```python
from build123d import *

# Parameters (mm, degrees)
CUT_EXTRUDE1_DEPTH      = 55.787705795
CUT_EXTRUDE1_DEPTH_BACK = 55.787705795
SKETCH2_R               = 11.8745
SKETCH2_R_2             = 3.175
CUT_EXTRUDE2_DEPTH      = 55.787705795
CUT_EXTRUDE2_DEPTH_BACK = 55.787705795
SKETCH3_R               = 3.175
CUT_EXTRUDE3_DEPTH      = 55.787705795
CUT_EXTRUDE3_DEPTH_BACK = 55.787705795
SKETCH4_R               = 3.175


with BuildPart() as part:
    # Sketch1 → Revolve1 (revolve)
    with BuildSketch(Plane.XY, mode=Mode.PRIVATE) as revolve1_sk:
        Polygon((0, 0), (36.5125, 0), (36.5125, 3.175), (38.1508, 3.175), (38.1508, 9.525), (0, 9.525), align=None)
    revolve(revolve1_sk.sketch.rotate(Axis((0, 0, 0), (0, 1, 0)), 90), axis=Axis((0, 0, 0), (0, 1, 0)))

    # Sketch2 → Cut-Extrude1 (cut, two sides: drawn at the far end of the back side and taken through both)
    with BuildSketch(Plane(origin=(0, 9.525, 0), x_dir=(1, 0, 0), z_dir=(0, 1, 0)).offset(-CUT_EXTRUDE1_DEPTH_BACK)):
        with Locations(Location((-12.7, 20.0152, 0), (0, 0, 270))):
            Circle(SKETCH2_R)
        with Locations(Location((12.7, 20.0152, 0), (0, 0, 270))):
            Circle(SKETCH2_R)
        with Locations(Location((0, 30.1752, 0), (0, 0, 270))):
            Circle(SKETCH2_R_2)
        with Locations(Location((0, 9.8552, 0), (0, 0, 270))):
            Circle(SKETCH2_R_2)
    extrude(amount=CUT_EXTRUDE1_DEPTH + CUT_EXTRUDE1_DEPTH_BACK, mode=Mode.SUBTRACT)

    # Sketch3 → Cut-Extrude2 (cut, two sides: drawn at the far end of the back side and taken through both)
    with BuildSketch(Plane(origin=(0, 9.525, 0), x_dir=(1, 0, 0), z_dir=(0, 1, 0)).offset(-CUT_EXTRUDE2_DEPTH_BACK)):
        with Locations(Location((-28.575, 0, 0), (0, 0, 270))):
            Circle(SKETCH3_R)
        with Locations(Location((28.575, 0, 0), (0, 0, 270))):
            Circle(SKETCH3_R)
    extrude(amount=CUT_EXTRUDE2_DEPTH + CUT_EXTRUDE2_DEPTH_BACK, mode=Mode.SUBTRACT)

    # Sketch4 → Cut-Extrude3 (cut, two sides: drawn at the far end of the back side and taken through both)
    with BuildSketch(Plane(origin=(0, 9.525, 0), x_dir=(1, 0, 0), z_dir=(0, 1, 0)).offset(-CUT_EXTRUDE3_DEPTH_BACK)):
        with Locations(Location((-15.875, -9.652, 0), (0, 0, 270))):
            Circle(SKETCH4_R)
        with Locations(Location((15.875, -9.652, 0), (0, 0, 270))):
            Circle(SKETCH4_R)
    extrude(amount=CUT_EXTRUDE3_DEPTH + CUT_EXTRUDE3_DEPTH_BACK, mode=Mode.SUBTRACT)


solid = part.part
```
Could you check a few things on this model? Use its own coordinates, in mm. A direction names the side the tool comes from. Give positions to 0.01 mm unless a question says otherwise; leave off trailing zeros. Loops run counter-clockwise (first coordinate to the right, second up) from the corner with the lowest first, then second, coordinate; pieces in that order, holes last. Notation, with made-up numbers: (45, 81) - (67, 81) arc R14 ccw to (67, 92) - close; hole circle Ø11 at (60.5, -20). An arc over 180 degrees is marked (long way). Use one line per item in the form item = value.
1. Thinking about a two-plate mould opening in X: for faces 1 (the face through (-25.427, 4.696, -0.413)), 2 (the face through (23.21, 6.39, 30.28)), 3 (the face through (-1, 9.525, 1)), which applies, released by +X, released by -X, zero draft, split by the parting line, or undercut?
Response values:
face_1 = undercut
face_2 = split by the parting line
face_3 = zero draft
2. I want a section at B-B (x = -9). Please give me the cut outline in (y, z) (3 decimals), and give its area (3 significant figures).
Response values:
outline = (0, -35.386) - (3.175, -35.386) - (3.175, -37.074) - (9.525, -37.074) - (9.525, -31.299) - (0, -31.299) - close; (0, -8.732) - (9.525, -8.732) - (9.525, 37.074) - (3.175, 37.074) - (3.175, 35.386) - (0, 35.386) - close
area = 481 mm²
3. I'm going to push flat-ended pins straight in: pin 1 Ø14 at (x, z) = (-12.7, -20.02) entering from +Y; pin 2 Ø4 at (y, z) = (3.5, 22.5) entering from +X; pin 3 Ø2 at (y, z) = (6, -13.5) entering from -X. Where does each tip first touch, or does it pass through?
Response values:
pin_1 = through
pin_2 = 32.18
pin_3 = -36.04
4. I need wall thicknesses on probe 1 along X at (y, z) = (9.25, -15); probe 2 along Z at (x, y) = (-15, 9.25); probe 3 along Z at (x, y) = (17.5, 1.5). Which ranges of each line are inside material? Lowest first, please.
Response values:
probe_1 = -35.08 to -23.46, -1.94 to 1.94, 23.46 to 35.08
probe_2 = -35.08 to -31.66, -8.37 to 6.6, 12.7 to 35.08
probe_3 = -32.05 to -30.88, -9.15 to 6.92, 12.38 to 32.05
5. I want a section at D-D (z = 18.5). Please give me the cut outline in (x, y) (3 decimals), and give its area (3 significant figures).
Response values:
outline = (-33.365, 3.175) - (-31.479, 3.175) - (-31.479, 0) - (31.479, 0) - (31.479, 3.175) - (33.365, 3.175) - (33.365, 9.525) - (-33.365, 9.525) - close
area = 624 mm²
6. On a 3-axis mill with a long thin cutter (end or side, diameter ignored), from which of +Z, -Z, +X, -X, +Y, -Y can I reach the whole of each face in a straight line? I mean faces 4 (the face through (25.476, 4.696, -0.688)), 5 (the face through (20, 3.175, 31)). Say none if no direction works.
Response values:
face_4 = +Y, -Y
face_5 = -Y
7. I want a section at A-A (z = 0). Give the number of separate pieces and of enclosed holes in the cut face, and give its area (3 significant figures).
Response values:
separate_pieces = 3
enclosed_holes = 0
area = 595 mm²
